Check sheet for the modelled part. Datum: model origin and axes. Units: mm. Face numbers are marked on the shaded views. Give positions to 0.01 mm unless a question says otherwise; leave off trailing zeros. Loops run counter-clockwise (first coordinate to the right, second up) from the corner with the lowest first, then second, coordinate; pieces in that order, holes last. Notation, with made-up numbers: (-38, 31) - (9, 31) arc R32 ccw to (9, 65) - close; hole circle Ø7 at (-19, -34). An arc over 180 degrees is marked (long way). Use one line per item in the form item = value.
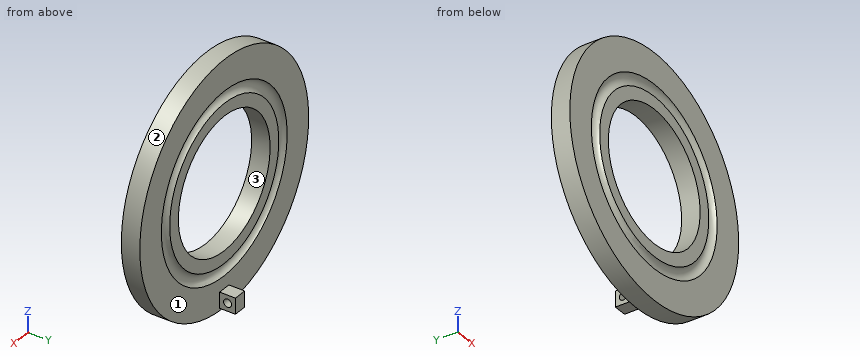
from build123d import *

# Parameters (mm, degrees)
CUT_EXTRUDE1_DEPTH      = 66.429351212
CUT_EXTRUDE1_DEPTH_BACK = 66.429351212
SKETCH4_R               = 25
SKETCH5_W               = 5
SKETCH5_H               = 6
BOSS_EXTRUDE1_DEPTH     = 13
CUT_EXTRUDE2_DEPTH      = 67.340033162
CUT_EXTRUDE2_DEPTH_BACK = 67.340033162
SKETCH6_R               = 1.5


with BuildPart() as part:
    # Sketch3 → Revolve1 (revolve)
    with BuildSketch(Plane.XY, mode=Mode.PRIVATE) as revolve1_sk:
        with BuildLine():
            Line((0, 0), (-29.729399859, 0))
            ThreePointArc((-29.729399859, 0), (-32, 1.825), (-34.270600141, 0))
            Line((-34.270600141, 0), (-46, 0))
            Line((-46, 0), (-46, 7))
            Line((-46, 7), (-34.270600141, 7))
            ThreePointArc((-34.270600141, 7), (-32, 5.175), (-29.729399859, 7))
            Line((-29.729399859, 7), (0, 7))
            Line((0, 7), (0, 0))
        make_face()
    revolve(revolve1_sk.sketch.rotate(Axis((0, 0, 0), (0, 1, 0)), 270), axis=Axis((0, 0, 0), (0, 1, 0)))

    # Sketch4 → Cut-Extrude1 (cut, two sides: drawn at the far end of the back side and taken through both)
    with BuildSketch(Plane(origin=(0, 7, 0), x_dir=(1, 0, 0), z_dir=(0, 1, 0)).offset(-CUT_EXTRUDE1_DEPTH_BACK)):
        with Locations(Location((0, 0, 0), (0, 0, 270))):
            Circle(SKETCH4_R)
    extrude(amount=CUT_EXTRUDE1_DEPTH + CUT_EXTRUDE1_DEPTH_BACK, mode=Mode.SUBTRACT)

    # Sketch5 → Boss-Extrude1 (add)
    with BuildSketch(Plane(origin=(0, 0, 0), x_dir=(1, 0, 0), z_dir=(0, 1, 0))):
        with Locations((0, 42)):
            Rectangle(SKETCH5_W, SKETCH5_H)
    extrude(amount=BOSS_EXTRUDE1_DEPTH)

    # Sketch6 → Cut-Extrude2 (cut, two sides: drawn at the far end of the back side and taken through both)
    with BuildSketch(Plane(origin=(0, 0, 0), x_dir=(0, 0, -1), z_dir=(1, 0, 0)).offset(-CUT_EXTRUDE2_DEPTH_BACK)):
        with Locations((42, 10)):
            Circle(SKETCH6_R)
    extrude(amount=CUT_EXTRUDE2_DEPTH + CUT_EXTRUDE2_DEPTH_BACK, mode=Mode.SUBTRACT)


solid = part.part
Item 1: Section check D-D on z = -42. Record the boundary of the cut face in (x, y).
Answer block:
outline = (-18.76, 0) - (18.76, 0) - (18.76, 7) - (2.5, 7) - (2.5, 8.5) - (-2.5, 8.5) - (-2.5, 7) - (-18.76, 7) - close; (-2.5, 11.5) - (2.5, 11.5) - (2.5, 13) - (-2.5, 13) - close
Item 2: Mould release check, pull along Z, two halves, no side actions. Record for the marked faces 1, 2 and 3: released by +Z, released by -Z, zero draft, split by the parting line, or undercut.
Answer block:
face_1 = zero draft
face_2 = split by the parting line
face_3 = undercut
Item 3: Section check B-B on y = 10. Record the boundary of the cut face in (x, z), then the cut area to 3 significant figures.
Answer block:
outline = (-2.5, -45) - (2.5, -45) - (2.5, -43.5) - (-2.5, -43.5) - close; (-2.5, -40.5) - (2.5, -40.5) - (2.5, -39) - (-2.5, -39) - close
area = 15.0 mm2
Item 4: Gauge pin test, flat ends, axial feed: P1, Ø3, axis at y = 10.5, z = -41.5, coming from the +X side; P2, Ø1, axis at x = 28, z = 1.5, coming from the +Y side; P3, Ø6, axis at y = 4.5, z = -15.5, coming from the -X side. Record the tip position at first contact, or that the pin passes through.
Answer block:
P1 = 2.5
P2 = 7
P3 = -44.27
Item 5: Thickness scan on L1, parallel to Z at x = -0.15, y = 10; L2, parallel to X at y = 3.5, z = 0; L3, parallel to X at y = 1.25, z = 17. Record the ranges inside material, lowest first.
Answer block:
L1 = -45 to -43.5, -40.5 to -39
L2 = -46 to -25, 25 to 46
L3 = -42.74 to -28.9, -25.29 to -18.33, 18.33 to 25.29, 28.9 to 42.74
Item 6: Section check A-A on x = 0. Record the boundary of the cut face in (y, z) (3 decimals).
Answer block:
outline = (0, -46) - (7, -46) - (7, -45) - (13, -45) - (13, -39) - (7, -39) - (7, -34.271) arc R2.325 cw to (7, -29.729) - (7, -25) - (0, -25) - (0, -29.729) arc R2.325 cw to (0, -34.271) - close; (0, 25) - (7, 25) - (7, 29.729) arc R2.325 cw to (7, 34.271) - (7, 46) - (0, 46) - (0, 34.271) arc R2.325 cw to (0, 29.729) - close; hole circle Ø3 at (10, -42)
Item 7: Section check C-C on z = 0. Record the boundary of the cut face in (x, y) (3 decimals), then the cut area to 3 significant figures.
Answer block:
outline = (-46, 0) - (-34.271, 0) arc R2.325 cw to (-29.729, 0) - (-25, 0) - (-25, 7) - (-29.729, 7) arc R2.325 cw to (-34.271, 7) - (-46, 7) - close; (25, 0) - (29.729, 0) arc R2.325 cw to (34.271, 0) - (46, 0) - (46, 7) - (34.271, 7) arc R2.325 cw to (29.729, 7) - (25, 7) - close
area = 269 mm2
